Input: part model. Units: mm. Frame: model coordinates. Round coordinates to 2 decimals unless told otherwise and drop trailing zeros. Order: outer loops, then holes, each group sorted by start corner. A loop starts at its lowest first (then second) coordinate and runs counter-clockwise, first axis right, second up. Notation, with made-up numbers: (50, 44.5) -> (95, 44.5) arc R8 cw to (95, 49.5) -> close; hole circle Ø9 at (71, 1.5). An arc over 180 degrees is marked (long way). Use a Markdown table: item, result.
from build123d import *

# Parameters (mm, degrees)
BOSS_EXTRUDE1_DEPTH = 11.4
SKETCH2_R           = 0.2
BOSS_EXTRUDE2_DEPTH = 3.2


with BuildPart() as part:
    # Sketch1 → Boss-Extrude1 (new body)
    with BuildSketch(Plane(origin=(0, 0, 0), x_dir=(1, 0, 0), z_dir=(0, 1, 0))):
        with BuildLine():
            Line((3.125, 0.561248608), (3.125, -0.561248608))
            ThreePointArc((3.125, -0.561248608), (-3.175, 0), (3.125, 0.561248608))
        make_face()
    extrude(amount=BOSS_EXTRUDE1_DEPTH)

    # Sketch2 → Boss-Extrude2 (add)
    with BuildSketch(Plane.XZ):
        with Locations((-1.27, 0)):
            Circle(SKETCH2_R)
        with Locations((1.27, 0)):
            Circle(SKETCH2_R)
    extrude(amount=BOSS_EXTRUDE2_DEPTH)


solid = part.part
1) Cut plane A-A on z = 0. Return loops of the section in (x, y) (3 decimals), and give its area (3 significant figures).
Results found:
| item | result |
|---|---|
| outline | (-3.175, 0) -> (-1.47, 0) -> (-1.47, -3.2) -> (-1.07, -3.2) -> (-1.07, 0) -> (1.07, 0) -> (1.07, -3.2) -> (1.47, -3.2) -> (1.47, 0) -> (3.125, 0) -> (3.125, 11.4) -> (-3.175, 11.4) -> close |
| area | 74.4 mm² |
2) Pull-direction query (Y, two-part tool) for faces 1 (the flat face through (3.125, 6, 0)), 2 (the flat face through (0, 11.4, 0)), 3 (the flat face through (0, 0, 0)); classes: +Y half, -Y half, draft (parallel to the pull), parting line (faces both ways), or undercut.
Results found:
| item | result |
|---|---|
| face 1 | draft |
| face 2 | +Y half |
| face 3 | -Y half |
3) Pin query (flat end, axial travel): pin 1 Ø1 at (y, z) = (5, -2) entering from -X; pin 2 Ø2 at (x, z) = (-2.5, -0.5) entering from -Y. Return the tip coordinate at first contact, or that it passes through.
Results found:
| item | result |
|---|---|
| pin 1 | stops at x = -2.8 |
| pin 2 | stops at y = 0 |
4) Cut plane B-B on y = -0.25. Return loops of the section in (x, z).
Results found:
| item | result |
|---|---|
| outline | circle Ø0.4 at (-1.27, 0); circle Ø0.4 at (1.27, 0) |
5) Line query: L1, parallel to Y at x = 2.25, z = 0.75; L2, parallel to Z at x = 2, y = 4; L3, parallel to Z at x = -0.5, y = 10.75. Output: solid intervals per line, ascending. Write a range as [from, to].
Results found:
| item | result |
|---|---|
| L1 | y = [0, 11.4] |
| L2 | z = [-2.47, 2.47] |
| L3 | z = [-3.14, 3.14] |
6) Cut plane C-C on x = 0. Return loops of the section in (y, z) (3 decimals).
Results found:
| item | result |
|---|---|
| outline | (0, -3.175) -> (11.4, -3.175) -> (11.4, 3.175) -> (0, 3.175) -> close |
7) Cut plane D-D on y = 3. Return loops of the section in (x, z) (3 decimals), and give its area (3 significant figures).
Results found:
| item | result |
|---|---|
| outline | (3.125, -0.561) -> (3.125, 0.561) arc R3.175 ccw (long way) to start |
| area | 31.6 mm² |
